Source: three-view drawing plus pictorial views. Frame: mm from the lowest corner of the part. Give positions to 0.01 mm unless a question says otherwise; leave off trailing zeros. Write each loop counter-clockwise with the first axis right and the second up, starting at its lowest first coordinate (ties: lowest second). Pieces come first, ordered by that corner, then holes. Notation, with made-up numbers: (68, -9) -> (126, -9) arc R22 ccw to (126, 26) -> close; hole circle Ø2 at (-16, 81). An arc over 180 degrees is marked (long way). Answer in a Markdown table with one row per item. Add a question column.
Item 1: Section query B-B on z = 0.6. State how many separate pieces and enclosed holes the cut face has, plus the area to 3 significant figures.
Item 2: First-contact query: P1, Ø2, axis at x = 16.75, y = 2.38, coming from the -Z side. Flat tip, straight axial feed; report the tip coordinate or a pass-through.
Item 3: Section query A-A on x = 16.75. Output: boundary loops of the cut face in (y, z) (1 decimal).
Item 4: Material intervals for probe 1 along Y at (x, z) = (16.75, 0.3) (1 decimal); probe 2 along X at (y, z) = (27.5, 0.3); probe 3 along Y at (x, z) = (4, 0.8) (1 decimal), sorted ascending. Write a range as from..to.
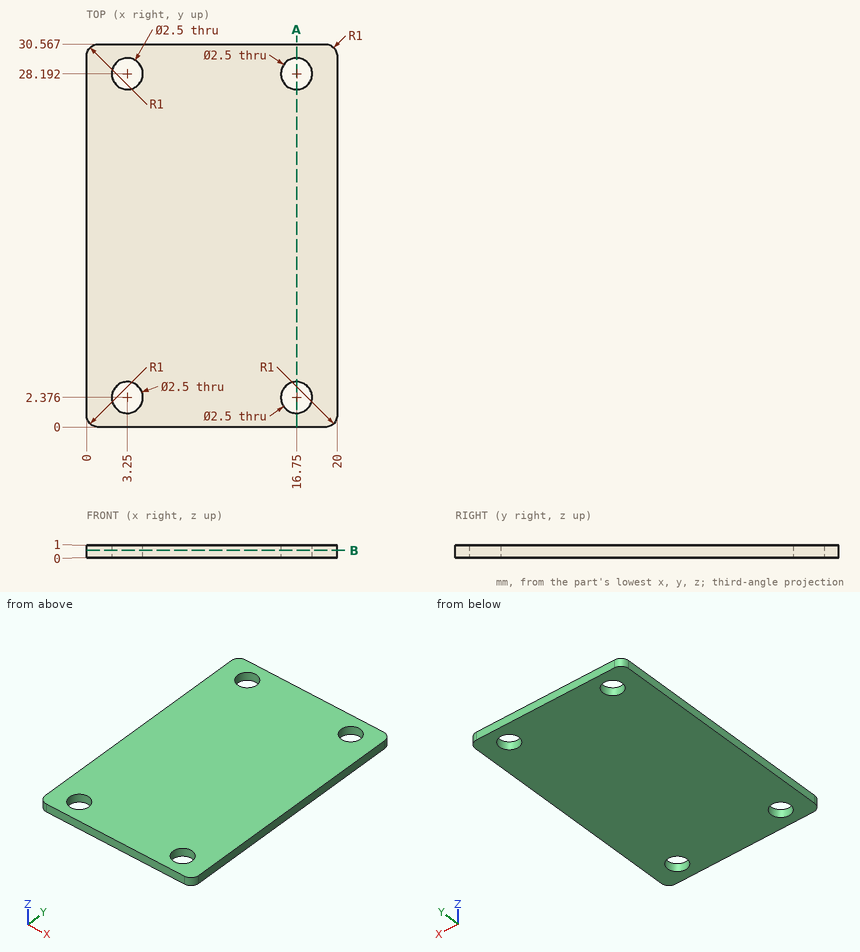
Findings below:
| question | item | result |
|---|---|---|
| 1 | separate pieces | 1 |
| 1 | enclosed holes | 4 |
| 1 | area | 591 mm^2 |
| 2 | P1 | passes through |
| 3 | outline | (0, 0) -> (1.1, 0) -> (1.1, 1) -> (0, 1) -> close; (3.6, 0) -> (26.9, 0) -> (26.9, 1) -> (3.6, 1) -> close; (29.4, 0) -> (30.6, 0) -> (30.6, 1) -> (29.4, 1) -> close |
| 4 | probe 1 | y = 0..1.1, 3.6..26.9, 29.4..30.6 |
| 4 | probe 2 | x = 0..2.21, 4.29..15.71, 17.79..20 |
| 4 | probe 3 | y = 0..1.4, 3.4..27.2, 29.2..30.6 |
